```python
from build123d import *

# Parameters (mm, degrees)
F1_DEPTH = 25
F2_DEPTH = 25
F3_DEPTH = 25
F4_DEPTH = 25
F5_DEPTH = 25


with BuildPart() as f1:
    # F0 (on Front) → F1 (new body)
    with BuildSketch(Plane.XZ):
        Polygon((-83.388145, 53.431101), (-103.388145, 53.431101), (-103.388145, -56.568899), (56.611855, -56.568899), (56.611855, -36.568899), align=None)
    extrude(amount=F1_DEPTH)

    # F0 (on Front) → F2 (join)
    with BuildSketch(Plane.XZ):
        Polygon((-83.388145, 53.431101), (-103.388145, 53.431101), (-103.388145, -56.568899), (56.611855, -56.568899), (56.611855, -36.568899), align=None)
    extrude(amount=F2_DEPTH)

    # F0 (on Front) → F3 (join)
    with BuildSketch(Plane.XZ):
        Polygon((-83.388145, 53.431101), (-103.388145, 53.431101), (-103.388145, -56.568899), (56.611855, -56.568899), (56.611855, -36.568899), align=None)
    extrude(amount=F3_DEPTH)

    # F0 (on Front) → F4 (join)
    with BuildSketch(Plane.XZ):
        Polygon((-83.388145, 53.431101), (-103.388145, 53.431101), (-103.388145, -56.568899), (56.611855, -56.568899), (56.611855, -36.568899), align=None)
    extrude(amount=F4_DEPTH)

    # F0 (on Front) → F5 (join)
    with BuildSketch(Plane.XZ):
        Polygon((-83.388145, 53.431101), (-103.388145, 53.431101), (-103.388145, -56.568899), (56.611855, -56.568899), (56.611855, -36.568899), align=None)
    extrude(amount=F5_DEPTH)


solid = f1.part
```
Work out the finished part from the listing and answer in its coordinate system (mm). Give positions to 0.01 mm unless a question says otherwise; leave off trailing zeros. Order: outer loops, then holes, each group sorted by start corner. A loop starts at its lowest first (then second) coordinate and runs counter-clockwise, first axis right, second up. Notation, with made-up numbers: M 3,83 L 59,83 A11 cw 59,97 Z; hole C 78,61 d5. An arc over 180 degrees is marked long. Return JSON: item names as keys, results as strings.
1) Section C-C, the plane z = 22 is taken. Write down the section's boundary in (x, y), plus the area to 3 significant figures.
Resolved:
{"outline": "M -103.39,-25 L -34.5,-25 L -34.5,0 L -103.39,0 Z", "area": "1,720 mm^2"}
2) Straight lines are drawn through the part: line 1 along Z through (x, y) = (-70.5, -1.25); line 2 along X through (y, z) = (-16.5, 2.5); line 3 along X through (y, z) = (-15.75, 26). For each, find the intervals that lie inside material, in ascending order. Write a range as [from, to].
Resolved:
{"line 1": "[-56.57, 45.15]", "line 2": "[-103.39, -4.16]", "line 3": "[-103.39, -40.72]"}
3) Section B-B, the plane x = 14 is taken. Write down the section's boundary in (y, z).
Resolved:
{"outline": "M -25,-56.57 L 0,-56.57 L 0,-9.18 L -25,-9.18 Z"}
4) Each of these flat-tipped pins is pushed along its axis until it touches: pin 1 (6 mm diameter, centred on x = -34.5, y = -16, fed in from +Z); pin 2 (6 mm diameter, centred on x = -4.5, y = -21, fed in from +Z). Where does it stop, or does it pass through?
Resolved:
{"pin 1": "z = 23.93", "pin 2": "z = 4.65"}
5) Section A-A, the plane y = -2 is taken. Write down the section's boundary in (x, z).
Resolved:
{"outline": "M -103.39,-56.57 L 56.61,-56.57 L 56.61,-36.57 L -83.39,53.43 L -103.39,53.43 Z"}
